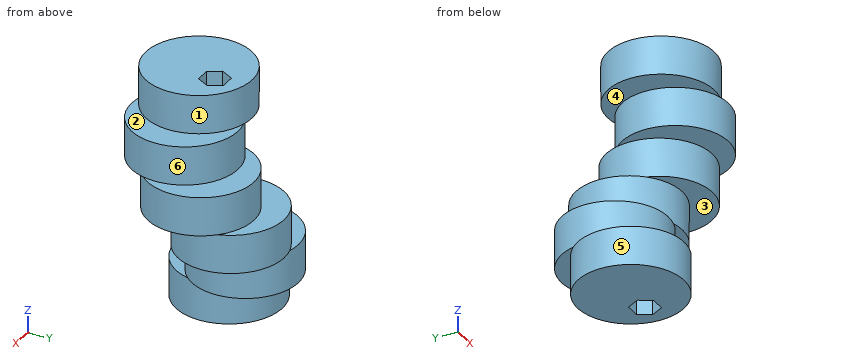
```python
from build123d import *

# Parameters (mm, degrees)
SKETCH1_R           = 11
BOSS_EXTRUDE1_DEPTH = 8
SKETCH3_R           = 11
BOSS_EXTRUDE2_DEPTH = 8
SKETCH4_R           = 11
BOSS_EXTRUDE4_DEPTH = 8
SKETCH5_R           = 11
BOSS_EXTRUDE5_DEPTH = 8
SKETCH6_R           = 11
BOSS_EXTRUDE6_DEPTH = 8
SKETCH8_R           = 11
BOSS_EXTRUDE7_DEPTH = 8
CUT_EXTRUDE1_DEPTH  = 48


with BuildPart() as part:
    # Sketch1 → Boss-Extrude1 (new body)
    with BuildSketch(Plane.XY):
        Circle(SKETCH1_R)
    extrude(amount=BOSS_EXTRUDE1_DEPTH)

    # Sketch3 → Boss-Extrude2 (add)
    with BuildSketch(Plane.XY.offset(8)):
        with Locations(Location((2.75, 4.763139721, 0), (0, 0, 164.477512186))):
            Circle(SKETCH3_R)
    extrude(amount=BOSS_EXTRUDE2_DEPTH)

    # Sketch4 → Boss-Extrude4 (add)
    with BuildSketch(Plane.XY.offset(16)):
        with Locations(Location((8.25, 4.763139721, 0), (0, 0, 255.522487814))):
            Circle(SKETCH4_R)
    extrude(amount=BOSS_EXTRUDE4_DEPTH)

    # Sketch5 → Boss-Extrude5 (add)
    with BuildSketch(Plane.XY.offset(24)):
        with Locations(Location((11, 0, 0), (0, 0, 195.522487814))):
            Circle(SKETCH5_R)
    extrude(amount=BOSS_EXTRUDE5_DEPTH)

    # Sketch6 → Boss-Extrude6 (add)
    with BuildSketch(Plane.XY.offset(32)):
        with Locations(Location((8.25, -4.763139721, 0), (0, 0, 135.522487814))):
            Circle(SKETCH6_R)
    extrude(amount=BOSS_EXTRUDE6_DEPTH)

    # Sketch8 → Boss-Extrude7 (add)
    with BuildSketch(Plane.XY.offset(40)):
        with Locations(Location((2.75, -4.763139721, 0), (0, 0, 284.477512186))):
            Circle(SKETCH8_R)
    extrude(amount=BOSS_EXTRUDE7_DEPTH)

    # Sketch9 → Cut-Extrude1 (cut)
    with BuildSketch(Plane.XY.offset(48)):
        Polygon((8.5, 0), (7, 2.598076211), (4, 2.598076211), (2.5, 0), (4, -2.598076211), (7, -2.598076211), align=None)
    extrude(amount=-CUT_EXTRUDE1_DEPTH, mode=Mode.SUBTRACT)


solid = part.part
```
Geometry: final body of the model. Coordinates: model frame, mm. Face numbers are marked on the shaded views. A direction names the side the tool comes from. Coordinates: 2 decimals unless noted, no trailing zeros. Order: outer loops, then holes, each group sorted by start corner. A loop starts at its lowest first (then second) coordinate and runs counter-clockwise, first axis right, second up. Notation, with made-up numbers: M 55,-23 L 111,-23 A28 cw 111,-3 Z; hole C -16.75,-28.5 d6. An arc over 180 degrees is marked long. Answer in a Markdown table with one row per item. Add a question column.
Q1. Section query C-C on y = 12. Return the cut outline in (x, z).
Q2. Reachability of the marked faces 4, 5 and 6 from +Z, -Z, +X, -X, +Y, -Y: full face, straight path, thin tool, end or side. Return the list, or none.
Q3. Mould query, pull axis Z, two halves, no side actions, for the marked faces 1, 2 and 3. Classes: released by +Z, released by -Z, zero draft, split by the parting line, or undercut.
Q4. Section query B-B on x = -4. Return the cut outline in (y, z).
Q5. Line query: L1, parallel to Z at x = 11.5, y = -0.5; L2, parallel to Z at x = 2.5, y = 12; L3, parallel to Y at x = 3, z = 11. Output: solid intervals per line, ascending.
Q6. Section query A-A on z = 14. Return the cut outline in (x, y).
Q7. Contact query for flat-ended pins moving along their axis: P1, Ø12, axis at y = -3, z = 39, coming from the -X side; P2, Ø2.5, axis at x = 5.5, z = 15.5, coming from the +Y side; P3, Ø8, axis at x = -4, z = 30.5, coming from the +Y side. Output: stop coordinate, or through.
Completed:
| question | item | result |
|---|---|---|
| 1 | outline | M -5.53,8 L 11.03,8 L 11.03,16 L 16.53,16 L 16.53,24 L -0.03,24 L -0.03,16 L -5.53,16 Z |
| 2 | face 4 | -X |
| 2 | face 5 | -Z |
| 2 | face 6 | none |
| 3 | face 1 | zero draft |
| 3 | face 2 | released by +Z |
| 3 | face 3 | undercut |
| 4 | outline | M -13.45,40 L 3.92,40 L 3.92,48 L -13.45,48 Z; M -10.25,0 L 10.25,0 L 10.25,8 L 13.45,8 L 13.45,16 L -3.92,16 L -3.92,8 L -10.25,8 Z |
| 5 | L1 | z = 8 to 48 |
| 5 | L2 | z = 8 to 24 |
| 5 | L3 | y = -6.23 to -0.87, 0.87 to 15.76 |
| 6 | outline | C 2.75,4.76 d22; hole M 2.5,0 L 4,-2.6 L 7,-2.6 L 8.5,0 L 7,2.6 L 4,2.6 Z |
| 7 | P1 | stops at x = -8.25 |
| 7 | P2 | stops at y = 15.66 |
| 7 | P3 | stops at y = 2.17 |
